Source: CAD feature listing. Evaluate the final solid. Frame: model axes, mm. A direction names the side the tool comes from. Give positions to 0.01 mm unless a question says otherwise; leave off trailing zeros. Order: outer loops, then holes, each group sorted by start corner. A loop starts at its lowest first (then second) coordinate and runs counter-clockwise, first axis right, second up.
from build123d import *

# Parameters (mm, degrees)
F0_R     = 10
F0_W     = 8
F0_H     = 40
F0_R_2   = 30
F1_DEPTH = 8
F2_R     = 40


with BuildPart() as f1:
    # F0 (on Front) → F1 (new body)
    with BuildSketch(Plane.XZ):
        with BuildLine():
            ThreePointArc((-118.825361, -51.870755), (-97.612157, -43.083959), (-88.825361, -21.870755))
            ThreePointArc((-88.825361, -21.870755), (-97.612157, -0.657552), (-118.825361, 8.129245))
            ThreePointArc((-118.825361, 8.129245), (-148.825361, -21.870755), (-118.825361, -51.870755))
        make_face()
        with Locations((-118.825361, -21.870755)):
            Circle(F0_R, mode=Mode.SUBTRACT)
        with BuildLine():
            ThreePointArc((-118.825361, 8.129245), (-97.612157, -0.657552), (-88.825361, -21.870755))
            ThreePointArc((-88.825361, -21.870755), (-97.612157, -43.083959), (-118.825361, -51.870755))
            Line((-118.825361, -51.870755), (121.535592, -53.234036))
            ThreePointArc((121.535592, -53.234036), (91.876372, -23.065815), (121.87589, 6.764034))
            ThreePointArc((121.87589, 6.764034), (80.764156, 34.521015), (51.912313, 74.871923))
            ThreePointArc((51.912313, 74.871923), (54.92108, 64.740607), (55.9365, 54.220856))
            ThreePointArc((55.9365, 54.220856), (-9.899421, 0.298849), (-49.793784, 75.467933))
            ThreePointArc((-49.793784, 75.467933), (-78.328518, 35.667172), (-118.825361, 8.129245))
        make_face()
        with Locations((-38.0635, -23.235966)):
            Rectangle(F0_W, F0_H, mode=Mode.SUBTRACT)
        with Locations((39.9365, -23.235966)):
            Rectangle(F0_W, F0_H, mode=Mode.SUBTRACT)
        with BuildLine():
            ThreePointArc((-48.154233, 79.022065), (-48.961587, 77.239269), (-49.793784, 75.467933))
            ThreePointArc((-49.793784, 75.467933), (-9.899421, 0.298849), (55.9365, 54.220856))
            ThreePointArc((55.9365, 54.220856), (54.92108, 64.740607), (51.912313, 74.871923))
            ThreePointArc((51.912313, 74.871923), (50.952881, 76.939321), (50.027233, 79.022065))
            ThreePointArc((50.027233, 79.022065), (0.9365, 109.220856), (-48.154233, 79.022065))
        make_face()
        with Locations((0.9365, 54.220856)):
            Circle(F0_R_2, mode=Mode.SUBTRACT)
        with BuildLine():
            ThreePointArc((121.87589, 6.764034), (91.876372, -23.065815), (121.535592, -53.234036))
            Line((121.535592, -53.234036), (121.87589, -53.235966))
            ThreePointArc((121.87589, -53.235966), (143.089093, -44.44917), (151.87589, -23.235966))
            ThreePointArc((151.87589, -23.235966), (143.089093, -2.022763), (121.87589, 6.764034))
        make_face()
        with Locations((121.87589, -23.235966)):
            Circle(F0_R, mode=Mode.SUBTRACT)
    extrude(amount=F1_DEPTH)

    # F2
    f2_edges = [f1.edges().sort_by_distance(p)[0] for p in [
        (-118.825361, -4, 8.129245),
        (121.87589, -4, 6.764034),
    ]]
    fillet(f2_edges, radius=F2_R)


solid = f1.part
1) Section query A-A on z = -6.5. Output: boundary loops of the cut face in (x, y), and give its area (3 significant figures).
Checks:
outline: (-144.59, -8) - (-42.06, -8) - (-42.06, 0) - (-144.59, 0) - close; (-34.06, -8) - (35.94, -8) - (35.94, 0) - (-34.06, 0) - close; (43.94, -8) - (146.77, -8) - (146.77, 0) - (43.94, 0) - close
area: 2,200 mm2
2) Reachability of faces 4 (the face through (1.786, -3.944, 109.214)), 5 (the face through (35.936, -4, -24)) from +Z, -Z, +X, -X, +Y, -Y: full face, straight path, thin tool, end or side. Return the list, or none.
Checks:
face 4: +Z, +Y, -Y
face 5: +Y, -Y
3) Section query C-C on z = 43.5. Output: boundary loops of the cut face in (x, y).
Checks:
outline: (-70.9, -8) - (-27.08, -8) - (-27.08, 0) - (-70.9, 0) - close; (28.96, -8) - (72.32, -8) - (72.32, 0) - (28.96, 0) - close
4) First-contact query: pin 1 Ø1.5 at (x, y) = (82.5, -2) entering from +Z; pin 2 Ø10 at (x, z) = (88, -24) entering from +Y; pin 3 Ø4 at (x, y) = (40.5, -5.5) entering from -Z; pin 4 Ø2.5 at (y, z) = (-2.5, -13.5) entering from -X. Flat tips, straight axial feed; report the tip coordinate or a pass-through.
Checks:
pin 1: stops at z = 33.57
pin 2: stops at y = 0
pin 3: stops at z = -52.79
pin 4: stops at x = -147.97
5) Section query D-D on y = -5. State how many separate pieces and enclosed holes the cut face has, and give its area (3 significant figures).
Checks:
separate pieces: 1
enclosed holes: 5
area: 26,100 mm2
6) Pull-direction query (X, two-part tool) for faces 1 (the face through (-1, 0, 11)), 2 (the face through (-148.776, -3.944, -23.591)), 3 (the face through (-5.567, -3.944, 24.934)); classes: +X half, -X half, draft (parallel to the pull), parting line (faces both ways), or undercut.
Checks:
face 1: draft
face 2: -X half
face 3: undercut
7) Ray query, L1, parallel to X at y = -4.25, z = 29; L2, parallel to X at y = -1, z = 73; L3, parallel to X at y = -7, z = -9.5. Return the intervals inside material, ascending.
Checks:
L1: x = -85.67 to -15.31, 17.18 to 86.78
L2: x = -51 to -22.46, 24.33 to 52.82
L3: x = -146.16 to -42.06, -34.06 to 35.94, 43.94 to 148.55
8) Section query B-B on x = -7.5. Output: boundary loops of the cut face in (y, z), and give its area (3 significant figures).
Checks:
outline: (-8, -52.5) - (0, -52.5) - (0, 25.43) - (-8, 25.43) - close; (-8, 83.01) - (0, 83.01) - (0, 108.57) - (-8, 108.57) - close
area: 828 mm2
